```python
from build123d import *

# Parameters (mm, degrees)
F0_R     = 38.1
F0_R_2   = 1.5875
F1_DEPTH = 22.86
F2_R     = 25.184471
F2_R_2   = 11.140075
F3_DEPTH = 15.24


with BuildPart() as f1:
    # F0 (on Right) → F1 (new body)
    with BuildSketch(Plane.YZ):
        Circle(F0_R)
        Circle(F0_R_2, mode=Mode.SUBTRACT)
    extrude(amount=F1_DEPTH)

    # F2 (on face) → F3 (cut)
    with BuildSketch(Plane.YZ.offset(22.86)):
        with Locations((-1.5875, 0)):
            Circle(F2_R)
        Circle(F2_R_2, mode=Mode.SUBTRACT)
    extrude(amount=-F3_DEPTH, mode=Mode.SUBTRACT)


solid = f1.part
```
Can you work these out from the model? Positions are in its coordinate system, mm. A direction names the side the tool comes from. Give positions to 0.01 mm unless a question says otherwise; leave off trailing zeros. Loops run counter-clockwise (first coordinate to the right, second up) from the corner with the lowest first, then second, coordinate; pieces in that order, holes last. Notation, with made-up numbers: M -3.5,2.25 L 47.5,2.25 A29 ccw 47.5,35.25 Z; hole C -9,12 d2. An arc over 180 degrees is marked long. One line per question, with ' | ' between items. Start each with the question number.
Q1. If I drill on line 1 (Z direction, x = 7, y = 0); line 2 (Y direction, x = 17.75, z = -3); line 3 (Z direction, x = 12.25, y = -2.5), over which ranges is the centre line in solid material (lowest first)? Write a range as from..to.
Q2. If we section it at D-D (y = -20.5): Please give me the cut outline in (x, z).
Q3. For pin 1 Ø3 at (x, z) = (3.5, 4) entering from -Y; pin 2 Ø3 at (y, z) = (0, 0) entering from -X; pin 3 Ø1 at (x, z) = (11.5, 22.5) entering from +Y; pin 4 Ø1.5 at (x, y) = (15.5, -19.5) entering from -Z, each with a flat end and sliding along its axis, tell me the tip position at first contact or that it passes through.
Q4. If we section it at A-A (z = 0): Please give me the cut outline in (x, y), plus the area to 3 significant figures.
Q5. If we mould it in two halves opening along Z, with no side actions, what happens to faces 3 (the flat face through (0, 8, 1)), 4 (the flat face through (7.62, -13, 0)), 5 (the cylindrical face through (11.27, -30.235, -23.183))? For each: +Z half, -Z half, draft (parallel to the pull), parting line (faces both ways), or undercut.
Q6. For faces 1 (the flat face through (22.86, 0, -2)), 2 (the cylindrical face through (15.347, 10.626, 3.346)), which set-ups out of +Z, -Z, +X, -X, +Y, -Y let a thin tool reach every point of the face, with its end or its side?
Q7. If we section it at B-B (y = 0): Please give me the cut outline in (x, z).
Q8. If we section it at C-C (x = 17.25): Please give me the cut outline in (y, z) (1 decimal), plus the area to 3 significant figures.
Computed:
1) line 1: z = -38.1..-1.59, 1.59..38.1 | line 2: y = -37.98..-26.59, -10.73..10.73, 23.42..37.98 | line 3: z = -38.02..-25.17, -10.86..10.86, 25.17..38.02
2) outline: M 0,-32.11 L 22.86,-32.11 L 22.86,-16.63 L 7.62,-16.63 L 7.62,16.63 L 22.86,16.63 L 22.86,32.11 L 0,32.11 Z
3) pin 1: stops at y = -38.02 | pin 2: passes through | pin 3: stops at y = 31.11 | pin 4: stops at z = -33.17
4) outline: M 0,-38.1 L 22.86,-38.1 L 22.86,-26.77 L 7.62,-26.77 L 7.62,-11.14 L 22.86,-11.14 L 22.86,-1.59 L 0,-1.59 Z; M 0,1.59 L 22.86,1.59 L 22.86,11.14 L 7.62,11.14 L 7.62,23.6 L 22.86,23.6 L 22.86,38.1 L 0,38.1 Z | area: 1,240 mm²
5) face 3: draft | face 4: undercut | face 5: parting line
6) face 1: +Z, -Z, +X, +Y, -Y | face 2: +X
7) outline: M 0,-38.1 L 22.86,-38.1 L 22.86,-25.13 L 7.62,-25.13 L 7.62,-11.14 L 22.86,-11.14 L 22.86,-1.59 L 0,-1.59 Z; M 0,1.59 L 22.86,1.59 L 22.86,11.14 L 7.62,11.14 L 7.62,25.13 L 22.86,25.13 L 22.86,38.1 L 0,38.1 Z
8) outline: C 0,0 d76.2; C 0,0 d22.3; hole C -1.6,0 d50.4; hole C 0,0 d3.2 | area: 2,950 mm²
